from build123d import *

# Parameters (mm, degrees)
SKETCH1_W                                    = 39.8018
SKETCH1_H                                    = 74.3712
BOSS_EXTRUDE1_SHOWN_IS_A_4_INCH_ACTUAT_DEPTH = 21.1074
FILLET1_RADIUS                               = 19.9009
FILLET1_LENGTH                               = 21.1074
CHAMFER1_SIZE                                = 7.7216
SKETCH2_R                                    = 19.1516
BOSS_EXTRUDE2_DEPTH                          = 74.5236
SKETCH3_R                                    = 6.2484
BOSS_EXTRUDE3_DEPTH                          = 3.3274
SKETCH4_W                                    = 17.8308
SKETCH4_H                                    = 17.8308
BOSS_EXTRUDE4_DEPTH                          = 19.0246
SKETCH5_R                                    = 2.9718
CUT_EXTRUDE1_DEPTH                           = 110.571496858
FILLET2_R                                    = 4.572
CHAMFER3_SIZE                                = 0.762
BODY_EXTRUDE_DEPTH                           = 164.08146
SKETCH7_R                                    = 9.9695
SHAFT_EXTRUDE_DEPTH                          = 100
SKETCH8_R                                    = 2.9845
CUT_EXTRUDE2_DEPTH                           = 12.7


with BuildPart() as part:
    # Sketch1 → Boss-Extrude1 - Shown is a 4 Inch Actuator (new body)
    with BuildSketch(Plane(origin=(0, 0, 0), x_dir=(1, 0, 0), z_dir=(0, 1, 0))):
        Rectangle(SKETCH1_W, SKETCH1_H)
    extrude(amount=BOSS_EXTRUDE1_SHOWN_IS_A_4_INCH_ACTUAT_DEPTH)

    # Fillet1: full round fillet: the end face becomes a half cylinder, R = half its width
    fillet1_face = Plane((0, 10.5537, 37.1856), x_dir=(0, 1, 0), z_dir=(0, 0, 1))  # on the end face: x along it, z out of the body
    fillet1_slab = fillet1_face.offset(-FILLET1_RADIUS / 2) * Box(FILLET1_LENGTH, 2 * FILLET1_RADIUS, FILLET1_RADIUS, mode=Mode.PRIVATE)  # the body's end, R deep
    fillet1_round = Plane((0, 10.5537, 17.2847), x_dir=(0, 0, 1), z_dir=(0, 1, 0)) * Cylinder(FILLET1_RADIUS, FILLET1_LENGTH, mode=Mode.PRIVATE)  # its axis R under the face
    add(fillet1_slab - fillet1_round, mode=Mode.SUBTRACT)

    # Chamfer1
    chamfer1_edges = [part.edges().sort_by_distance(p)[0] for p in [
        (-19.9009, 10.5537, -37.1856),
        (19.9009, 10.5537, -37.1856),
    ]]
    chamfer(chamfer1_edges, length=CHAMFER1_SIZE)

    # Sketch2 → Boss-Extrude2 (add)
    with BuildSketch(Plane(origin=(0, 21.1074, 0), x_dir=(1, 0, 0), z_dir=(0, 1, 0))):
        with Locations(Location((0, -17.2847, 0), (0, 0, 270))):
            Circle(SKETCH2_R)
    extrude(amount=BOSS_EXTRUDE2_DEPTH)

    # Sketch3 → Boss-Extrude3 (add)
    with BuildSketch(Plane(origin=(0, 95.631, 0), x_dir=(1, 0, 0), z_dir=(0, 1, 0))):
        with Locations(Location((0, -17.2847, 0), (0, 0, 270))):
            Circle(SKETCH3_R)
    extrude(amount=BOSS_EXTRUDE3_DEPTH)

    # Sketch4 → Boss-Extrude4 (add)
    with BuildSketch(Plane.XZ):
        with Locations((0, -17.6022)):
            Rectangle(SKETCH4_W, SKETCH4_H)
    extrude(amount=BOSS_EXTRUDE4_DEPTH)

    # Sketch5 → Cut-Extrude1 (cut, through all)
    with BuildSketch(Plane(origin=(8.9154, 0, 0), x_dir=(0, 0, -1), z_dir=(1, 0, 0))):
        with Locations((17.6022, -9.1694)):
            Circle(SKETCH5_R)
    extrude(amount=-CUT_EXTRUDE1_DEPTH, mode=Mode.SUBTRACT)

    # Fillet2
    fillet2_edges = [part.edges().sort_by_distance(p)[0] for p in [
        (8.9154, -9.5123, -26.5176),
        (8.9154, -9.5123, -8.6868),
        (-8.9154, -9.5123, -8.6868),
        (-8.9154, -9.5123, -26.5176),
    ]]
    fillet(fillet2_edges, radius=FILLET2_R)

    # Chamfer3
    chamfer3_edges = [part.edges().sort_by_distance(p)[0] for p in [
        (0, -19.0246, -26.5176),
        (-8.9154, -19.0246, -17.6022),
        (8.9154, -19.0246, -17.6022),
        (0, -19.0246, -8.6868),
        (7.576292204, -19.0246, -10.025907796),
        (7.576292204, -19.0246, -25.178492204),
        (-7.576292204, -19.0246, -10.025907796),
        (-7.576292204, -19.0246, -25.178492204),
    ]]
    chamfer(chamfer3_edges, length=CHAMFER3_SIZE)

    # Sketch6 → Body Extrude (add)
    with BuildSketch(Plane(origin=(0, 21.1074, 0), x_dir=(1, 0, 0), z_dir=(0, 1, 0))):
        with BuildLine():
            Line((0, 37.1856), (-10.3378, 37.1856))
            Line((-10.3378, 37.1856), (-14.428797676, 21.257258339))
            ThreePointArc((-14.428797676, 21.257258339), (0, 2.6543), (14.428797676, 21.257258339))
            Line((14.428797676, 21.257258339), (10.3378, 37.1856))
            Line((10.3378, 37.1856), (0, 37.1856))
        make_face()
    extrude(amount=BODY_EXTRUDE_DEPTH)

    # Sketch7 → Shaft Extrude (add)
    with BuildSketch(Plane(origin=(0, 185.18886, 0), x_dir=(1, 0, 0), z_dir=(0, 1, 0))):
        with Locations(Location((0, 17.5514, 0), (0, 0, 270))):
            Circle(SKETCH7_R)
    extrude(amount=SHAFT_EXTRUDE_DEPTH)

    # Sketch8 → Cut-Extrude2 (cut, symmetric)
    with BuildSketch(Plane(origin=(0, 0, 0), x_dir=(0, 0, -1), z_dir=(1, 0, 0))):
        with Locations((17.5514, 276.08296)):
            Circle(SKETCH8_R)
    extrude(amount=CUT_EXTRUDE2_DEPTH, both=True, mode=Mode.SUBTRACT)


solid = part.part
The model under review builds one solid part; all positions refer to its coordinate system, in mm. A direction names the side the tool comes from. Coordinates: 2 decimals unless noted, no trailing zeros. Order: outer loops, then holes, each group sorted by start corner. A loop starts at its lowest first (then second) coordinate and runs counter-clockwise, first axis right, second up. Notation, with made-up numbers: (64.25, -21) -> (79.25, -21) arc R18 ccw to (79.25, 8) -> close; hole circle Ø6 at (-16.5, 69.5). An arc over 180 degrees is marked (long way). Answer in a Markdown table with one row per item.
(1) Consider section D-D (y = 122.5). Write out the cut boundary in (x, z).
Answers:
| item | result |
|---|---|
| outline | (-14.43, -21.26) -> (-10.34, -37.19) -> (10.34, -37.19) -> (14.43, -21.26) arc R14.9 ccw (long way) to start |
(2) The part is to be moulded in two halves that separate along Z. For faces 6 (the cylindrical face through (0.14, 273.17, -16.9)), 7 (the flat face through (15.986, 10.406, -33.379)), 8 (the flat face through (0, 0, -1)), say which applies: +Z half, -Z half, draft (parallel to the pull), parting line (faces both ways), or undercut.
Answers:
| item | result |
|---|---|
| face 6 | undercut |
| face 7 | -Z half |
| face 8 | draft |
(3) Consider section B-B (x = 0). Write out the cut boundary in (y, z).
Answers:
| item | result |
|---|---|
| outline | (-19.02, -25.76) -> (-18.26, -26.52) -> (0, -26.52) -> (0, -37.19) -> (185.19, -37.19) -> (185.19, -27.52) -> (285.19, -27.52) -> (285.19, -7.58) -> (185.19, -7.58) -> (185.19, -2.65) -> (21.11, -2.65) -> (21.11, -1.87) -> (95.63, -1.87) -> (95.63, 11.04) -> (98.96, 11.04) -> (98.96, 23.53) -> (95.63, 23.53) -> (95.63, 36.44) -> (21.11, 36.44) -> (21.11, 37.19) -> (0, 37.19) -> (0, -8.69) -> (-18.26, -8.69) -> (-19.02, -9.45) -> close; hole circle Ø5.94 at (-9.17, -17.6); hole circle Ø5.97 at (276.08, -17.55) |
(4) Consider section C-C (z = 29.5). Write out the cut boundary in (x, y), plus the area to 3 significant figures.
Answers:
| item | result |
|---|---|
| outline | (-15.71, 0) -> (15.71, 0) -> (15.71, 21.11) -> (14.75, 21.11) -> (14.75, 95.63) -> (-14.75, 95.63) -> (-14.75, 21.11) -> (-15.71, 21.11) -> close |
| area | 2,860 mm² |
(5) Machinability: for faces 1 (the cylindrical face through (-0.38, 102, -2.66)), 2 (the flat face through (0, 98.958, 17)), 3 (the flat face through (-12.355, 102, -29.333)), 4 (the flat face through (12.41, 102, -29.11)), 5 (the flat face through (0, -9, -8.687)), which of the approach directions +Z, -Z, +X, -X, +Y, -Y give a long, thin tool a straight path to every point of the face, cutting with its end or side? Answer none if there is none.
Answers:
| item | result |
|---|---|
| face 1 | +Y |
| face 2 | +Z, +X, -X, +Y |
| face 3 | -Z, -X, +Y |
| face 4 | -Z, +X, +Y |
| face 5 | +Z, +X, -X, -Y |
(6) Wall thickness on line 1 along Y through (x, z) = (0, -18); line 2 along Y through (x, z) = (-1.5, -19); line 3 along X through (y, z) = (167, -6.5): over which ranges is each line inside the solid? List them lowest first.
Answers:
| item | result |
|---|---|
| line 1 | -19.02 to -12.11, -6.22 to 273.13, 279.03 to 285.19 |
| line 2 | -19.02 to -11.79, -6.55 to 273.47, 278.69 to 285.19 |
| line 3 | -9.99 to 9.99 |
(7) Insertion check: pin 1 (1 mm diameter, centred on x = 11.5, z = 25.5, fed in from +Y); pin 2 (9.5 mm diameter, centred on y = -11.5, z = -19.5, fed in from -X); pin 3 (7 mm diameter, centred on y = 276.08, z = -17.55, fed in from +X); pin 4 (3.5 mm diameter, centred on y = -9.17, z = -17.6, fed in from +X). Each pin has a flat end and moves straight along its axis. Give the tip position at first contact, or say it passes through.
Answers:
| item | result |
|---|---|
| pin 1 | y = 95.63 |
| pin 2 | x = -8.92 |
| pin 3 | x = 9.97 |
| pin 4 | through |
(8) Consider section A-A (y = 57). Write out the cut boundary in (x, z).
Answers:
| item | result |
|---|---|
| outline | circle Ø38.3 at (0, 17.28); (-14.43, -21.26) -> (-10.34, -37.19) -> (10.34, -37.19) -> (14.43, -21.26) arc R14.9 ccw (long way) to start |
